Source: CAD feature listing. Evaluate the final solid. Frame: model axes, mm. Face numbers are marked on the shaded views. A direction names the side the tool comes from. Coordinates: 2 decimals unless noted, no trailing zeros. Order: outer loops, then holes, each group sorted by start corner. A loop starts at its lowest first (then second) coordinate and runs counter-clockwise, first axis right, second up.
```python
from build123d import *

# Parameters (mm, degrees)
SKETCH1_W           = 300
SKETCH1_H           = 316
BOSS_EXTRUDE1_DEPTH = 300
FILLET1_R           = 50
SHELL1_T            = -40


with BuildPart() as part:
    # Sketch1 → Boss-Extrude1 (new body)
    with BuildSketch(Plane(origin=(0, 0, 0), x_dir=(1, 0, 0), z_dir=(0, 1, 0))):
        Rectangle(SKETCH1_W, SKETCH1_H)
    extrude(amount=BOSS_EXTRUDE1_DEPTH)

    # Fillet1
    fillet1_edges = [part.edges().sort_by_distance(p)[0] for p in [
        (-150, 150, -158),
        (150, 150, -158),
        (150, 150, 158),
        (-150, 150, 158),
    ]]
    fillet(fillet1_edges, radius=FILLET1_R)

    # Shell1
    shell1_openings = [part.faces().sort_by_distance(p)[0] for p in [
        (0, 300, 0),
        (0, 0, 0),
    ]]
    offset(amount=SHELL1_T, openings=shell1_openings, kind=Kind.INTERSECTION)


solid = part.part
```
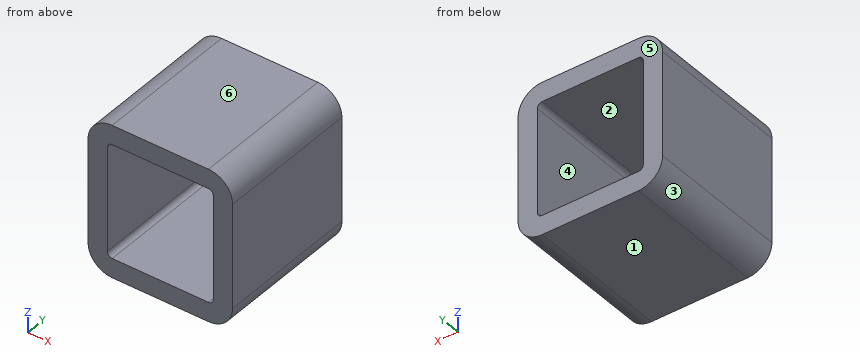
Q1. Pull-direction query (Z, two-part tool) for the marked faces 3, 4, 5 and 6; classes: pulls with the +Z half, pulls with the -Z half, needs draft (parallel to the pull), parting line crosses it, or undercut.
Solutions:
face 3: pulls with the -Z half
face 4: undercut
face 5: needs draft
face 6: pulls with the +Z half
Q2. Section query B-B on y = 277. Output: boundary loops of the cut face in (x, z), plus the area to 3 significant figures.
Solutions:
outline: (-150, -108) arc R50 ccw to (-100, -158) - (100, -158) arc R50 ccw to (150, -108) - (150, 108) arc R50 ccw to (100, 158) - (-100, 158) arc R50 ccw to (-150, 108) - close; hole (-110, -108) arc R10 ccw to (-100, -118) - (100, -118) arc R10 ccw to (110, -108) - (110, 108) arc R10 ccw to (100, 118) - (-100, 118) arc R10 ccw to (-110, 108) - close
area: 40,800 mm2
Q3. Set-up query: the marked faces 1 and 2. Return all of +Z, -Z, +X, -X, +Y, -Y with unobstructed straight access to the full face (end or side cutting, diameter ignored); none if empty.
Solutions:
face 1: -Z, +X, -X, +Y, -Y
face 2: +Y, -Y
Q4. Section query C-C on x = -30. Output: boundary loops of the cut face in (y, z), plus the area to 3 significant figures.
Solutions:
outline: (0, -158) - (300, -158) - (300, -118) - (0, -118) - close; (0, 118) - (300, 118) - (300, 158) - (0, 158) - close
area: 24,000 mm2
Q5. Section query D-D on x = 130. Output: boundary loops of the cut face in (y, z).
Solutions:
outline: (0, -148) - (300, -148) - (300, 148) - (0, 148) - close
Q6. Section query A-A on z = 102.5. Output: boundary loops of the cut face in (x, y), plus the area to 3 significant figures.
Solutions:
outline: (-150, 0) - (-110, 0) - (-110, 300) - (-150, 300) - close; (110, 0) - (150, 0) - (150, 300) - (110, 300) - close
area: 24,000 mm2
Q7. Material intervals for line 1 along X through (y, z) = (258, 53); line 2 along Z through (x, y) = (-59, 227); line 3 along X through (y, z) = (235.5, -109), sorted ascending.
Solutions:
line 1: x = -150 to -110, 110 to 150
line 2: z = -158 to -118, 118 to 158
line 3: x = -149.99 to -109.95, 109.95 to 149.99
